Print and shaded views of the part. All mm, measured from the part's lowest x, y and z. Coordinates: 2 decimals unless noted, no trailing zeros. Loops run counter-clockwise (first coordinate to the right, second up) from the corner with the lowest first, then second, coordinate; pieces in that order, holes last. Notation, with made-up numbers: (79.25, 77.5) -> (110.25, 77.5) arc R33 cw to (110.25, 115.5) -> close; hole circle Ø3 at (63, -37.75). An arc over 180 degrees is marked (long way). One line per item, written item: value. Start each with the question number.
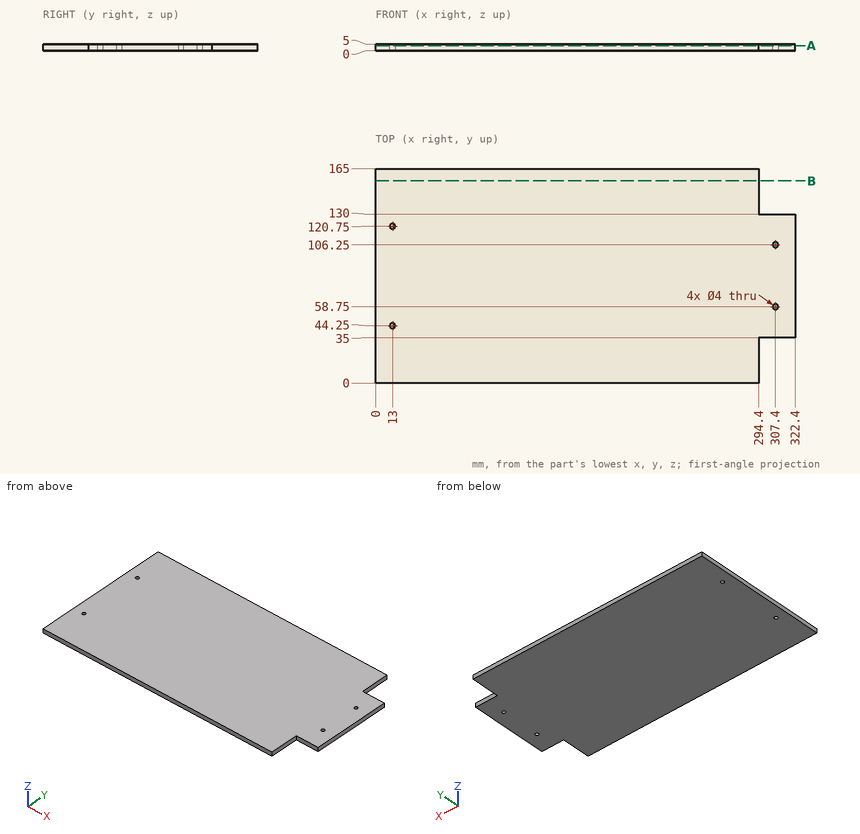
1) Probe line 1 (Y direction, x = 307.4, z = 3.1); line 2 (Y direction, x = 13, z = 3.85); line 3 (X direction, y = 7, z = 3.3). List the from-to ranges inside material, lowest first. Write a range as from..to.
2) Slice it at A-A (z = 3.8). Give the cut face in (x, y), then the cut area to 3 significant figures.
3) Slice it at B-B (y = 155.5). Give the cut face in (x, z).
Check sheet entries:
1. line 1: y = 35..56.75, 60.75..104.25, 108.25..130
1. line 2: y = 0..42.25, 46.25..118.75, 122.75..165
1. line 3: x = 0..294.4
2. outline: (0, 0) -> (294.4, 0) -> (294.4, 35) -> (322.4, 35) -> (322.4, 130) -> (294.4, 130) -> (294.4, 165) -> (0, 165) -> close; hole circle Ø4 at (13, 44.25); hole circle Ø4 at (13, 120.75); hole circle Ø4 at (307.4, 58.75); hole circle Ø4 at (307.4, 106.25)
2. area: 51,200 mm^2
3. outline: (0, 0) -> (294.4, 0) -> (294.4, 5) -> (0, 5) -> close
